Could you check a few things on this model? Use its own coordinates, in mm. A direction names the side the tool comes from. Coordinates: 2 decimals unless noted, no trailing zeros. Loops run counter-clockwise (first coordinate to the right, second up) from the corner with the lowest first, then second, coordinate; pieces in that order, holes last. Notation, with made-up numbers: (-37.5, -0.5) - (-15.5, -0.5) arc R8 ccw to (-15.5, 11.5) - close; hole circle Ø7 at (68, 0.5). An arc over 180 degrees is marked (long way). One line per item, written item: value. Start each with the question number.
(1) If we mould it in two halves opening along Y, with no side actions, what happens to faces 1 (the face through (2.96, 39.84, 24.19)), 2 (the face through (2.96, 15.33, 23.43)), 3 (the face through (6, 10, 5))? For each: pulls with the +Y half, pulls with the -Y half, needs draft (parallel to the pull), parting line crosses it, or undercut.
(2) If I drill on line 1 along Z through (x, y) = (4.55, 22); line 2 along Y through (x, z) = (5.7, -1); line 3 along Y through (x, z) = (1, 13), over which ranges is the centre line in solid material (lowest first)? Write a range as from..to.
(3) If we section it at A-A on z = 14.5: Write out the boundary of the cut face in (x, y), then the cut area to 3 significant figures.
(4) On a 3-axis mill with a long thin cutter (end or side, diameter ignored), from which of +Z, -Z, +X, -X, +Y, -Y can I reach the whole of each face in a straight line? I mean faces 4 (the face through (3, -4, 8.75)), 5 (the face through (3, -8.75, 1)), 6 (the face through (2.96, 12.39, 3.75)). Say none if no direction works.
(5) If we section it at D-D on y = 32: Write out the boundary of the cut face in (x, z), then the cut area to 3 significant figures.
(6) If we section it at C-C on y = 2: Write out the boundary of the cut face in (x, z).
(7) I'm going to push flat-ended pins straight in: P1, Ø8, axis at y = -4, z = 7, coming from the +X side; P2, Ø1.8, axis at x = 3, y = -4, coming from the -Z side; P3, Ø1, axis at x = 3.5, y = 9, coming from the +Z side; P4, Ø2, axis at x = 4.5, z = 1.5, coming from the +Y side. Where does each tip first touch, or does it pass through?
(8) If we section it at B-B on x = 1.65: Write out the boundary of the cut face in (y, z).
```python
from build123d import *

# Parameters (mm, degrees)
F1_DEPTH = 6


with BuildPart() as f1:
    # F0 (on Right) → F1 (new body)
    with BuildSketch(Plane.YZ):
        with BuildLine():
            ThreePointArc((0, 8.75), (6.187184, -6.187184), (-8.75, 0))
            Line((-8.75, 0), (-8.75, 2.75))
            Line((-8.75, 2.75), (-10.606602, 2.75))
            ThreePointArc((-10.606602, 2.75), (-11.253598, 2.512493), (-11.593262, 1.912791))
            ThreePointArc((-11.593262, 1.912791), (-11.739513, -0.496329), (-11.39044, -2.884507))
            Line((-11.39044, -2.884507), (-9.624207, -9.859066))
            ThreePointArc((-9.624207, -9.859066), (-9.323883, -10.35677), (-8.797476, -10.603346))
            Line((-8.797476, -10.603346), (-1.676351, -11.629804))
            Line((-1.676351, -11.629804), (5.599694, -12.678593))
            ThreePointArc((5.599694, -12.678593), (6.067344, -12.634542), (6.463292, -12.38183))
            Line((6.463292, -12.38183), (16.489511, -1.951659))
            Line((16.489511, -1.951659), (40.04656, 22.554495))
            ThreePointArc((40.04656, 22.554495), (40.229484, 22.81966), (40.318611, 23.129224))
            Line((40.318611, 23.129224), (40.327941, 23.207551))
            ThreePointArc((40.327941, 23.207551), (39.824234, 24.197961), (38.716454, 24.11161))
            Line((38.716454, 24.11161), (13.11122, 3.95707))
            ThreePointArc((13.11122, 3.95707), (12.374434, 3.749868), (11.706934, 4.124342))
            Line((11.706934, 4.124342), (9.232906, 7.267458))
            Line((9.232906, 7.267458), (6.758877, 10.410575))
            ThreePointArc((6.758877, 10.410575), (6.551676, 11.147362), (6.926149, 11.814862))
            Line((6.926149, 11.814862), (25.45937, 26.402838))
            ThreePointArc((25.45937, 26.402838), (25.803521, 27.459339), (24.959142, 28.181598))
            Line((24.959142, 28.181598), (24.854219, 28.194096))
            ThreePointArc((24.854219, 28.194096), (24.556198, 28.184829), (24.274156, 28.088108))
            Line((24.274156, 28.088108), (6.135427, 18.644765))
            ThreePointArc((6.135427, 18.644765), (2.099072, 16.297577), (-1.700732, 13.584103))
            Line((-1.700732, 13.584103), (-6.66306, 9.678126))
            Line((-6.66306, 9.678126), (-7.842194, 8.75))
            Line((-7.842194, 8.75), (0, 8.75))
        make_face()
        with BuildLine():
            ThreePointArc((-6.66306, 9.678126), (-7.267458, 9.232906), (-7.842194, 8.75))
            Line((-7.842194, 8.75), (-6.66306, 9.678126))
        make_face()
    extrude(amount=F1_DEPTH)


solid = f1.part
```
Values:
1. face 1: undercut
1. face 2: pulls with the -Y half
1. face 3: needs draft
2. line 1: z = 3.78..10.95, 23.68..26.9
2. line 2: y = -11.71..-8.69, 8.69..17.4
2. line 3: y = -2.44..8.43, 24.6..30.86
3. outline: (0, -0.5) - (6, -0.5) - (6, 10.34) - (0, 10.34) - close; (0, 26.51) - (6, 26.51) - (6, 32.3) - (0, 32.3) - close
3. area: 99.8 mm2
4. face 4: +X, -X, -Y
4. face 5: +Z, +X, -X
4. face 6: +X, -X
5. outline: (0, 14.18) - (6, 14.18) - (6, 18.82) - (0, 18.82) - close
5. area: 27.8 mm2
6. outline: (0, -12.16) - (6, -12.16) - (6, -8.52) - (0, -8.52) - close; (0, 8.52) - (6, 8.52) - (6, 16.23) - (0, 16.23) - close
7. P1: stops at x = 6
7. P2: stops at z = -11.42
7. P3: stops at z = 20.4
7. P4: stops at y = 20.77
8. outline: (-11.59, 1.91) arc R11.75 ccw to (-11.39, -2.88) - (-9.62, -9.86) arc R1 ccw to (-8.8, -10.6) - (5.6, -12.68) arc R1 ccw to (6.46, -12.38) - (40.05, 22.55) arc R1 ccw to (40.32, 23.13) - (40.33, 23.21) arc R1 ccw to (38.72, 24.11) - (13.11, 3.96) arc R1 cw to (11.71, 4.12) - (6.76, 10.41) arc R1 cw to (6.93, 11.81) - (25.46, 26.4) arc R1 ccw to (24.96, 28.18) - (24.85, 28.19) arc R1 ccw to (24.27, 28.09) - (6.14, 18.64) arc R50 ccw to (-1.7, 13.58) - (-6.66, 9.68) arc R11.75 ccw to (-7.84, 8.75) - (0, 8.75) arc R8.75 cw (long way) to (-8.75, 0) - (-8.75, 2.75) - (-10.61, 2.75) arc R1 ccw to start
